Answer from the drawing. Dimensions are ordinates in mm from the lowest x, y and z of the part. Give positions to 0.01 mm unless a question says otherwise; leave off trailing zeros. Order: outer loops, then holes, each group sorted by start corner. A loop starts at its lowest first (then second) coordinate and runs counter-clockwise, first axis right, second up. Notation, with made-up numbers: (-10, 18.25) - (47, 18.25) arc R32 ccw to (47, 52.25) - close; hole circle Ø9 at (76, -18.75). An arc over 180 degrees is marked (long way). Write each question's results on one line, items separated by ' | '.
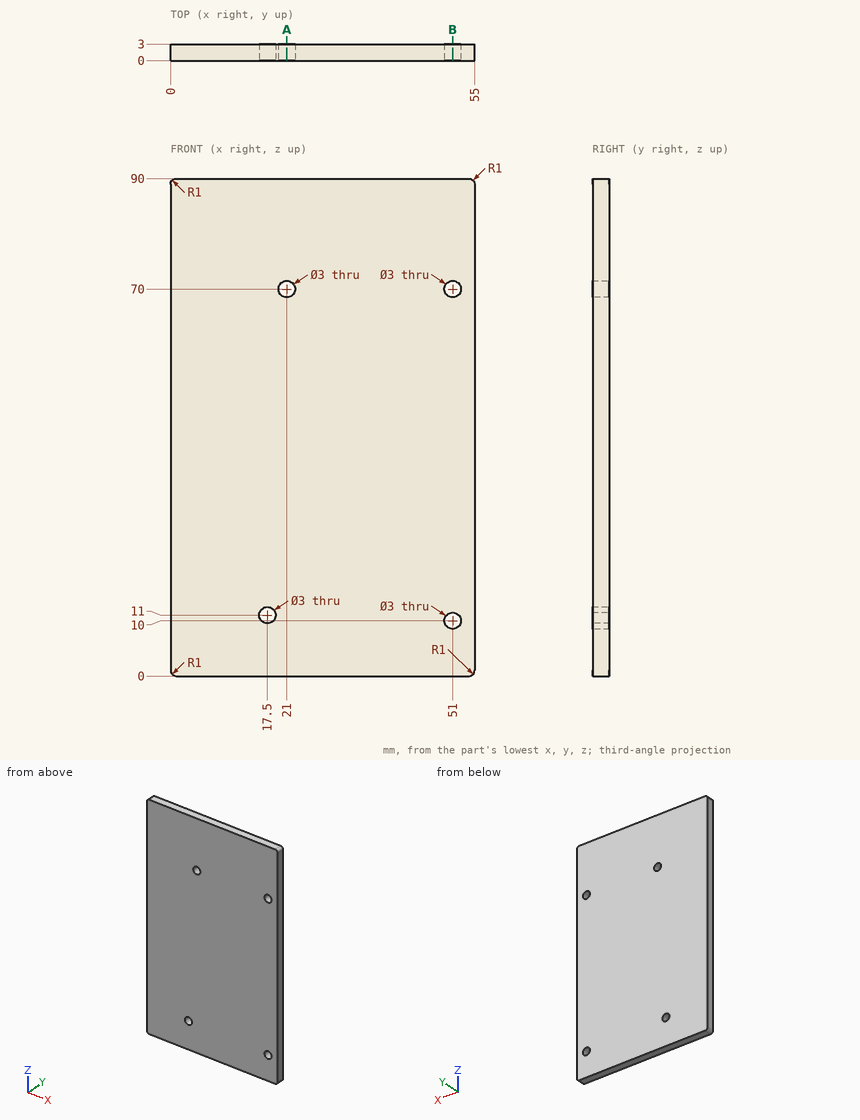
(1) Section B-B (x = 51) is taken. Give the vertices of the cut face in (y, z).
Conclusion:
outline: (0, 0) - (3, 0) - (3, 8.5) - (0, 8.5) - close; (0, 11.5) - (3, 11.5) - (3, 68.5) - (0, 68.5) - close; (0, 71.5) - (3, 71.5) - (3, 90) - (0, 90) - close
(2) This flat-tipped pin is pushed along its axis until it touches: pin 1 (2.5 mm diameter, centred on x = 51, z = 10, fed in from -Y). Where does it stop, or does it pass through?
Conclusion:
pin 1: through
(3) Section A-A (x = 21) is taken. Give the vertices of the cut face in (y, z).
Conclusion:
outline: (0, 0) - (3, 0) - (3, 68.5) - (0, 68.5) - close; (0, 71.5) - (3, 71.5) - (3, 90) - (0, 90) - close
(4) Consider probe 1 along X at (y, z) = (1.7, 70); probe 2 along X at (y, z) = (1.5, 11); probe 3 along Z at (x, y) = (50, 2.2). Determine where each line is inside the solid, lowest interval first. Write a range as [from, to].
Conclusion:
probe 1: [0, 19.5], [22.5, 49.5], [52.5, 55] | probe 2: [0, 16], [19, 49.88], [52.12, 55] | probe 3: [0, 8.88], [11.12, 68.88], [71.12, 90]
